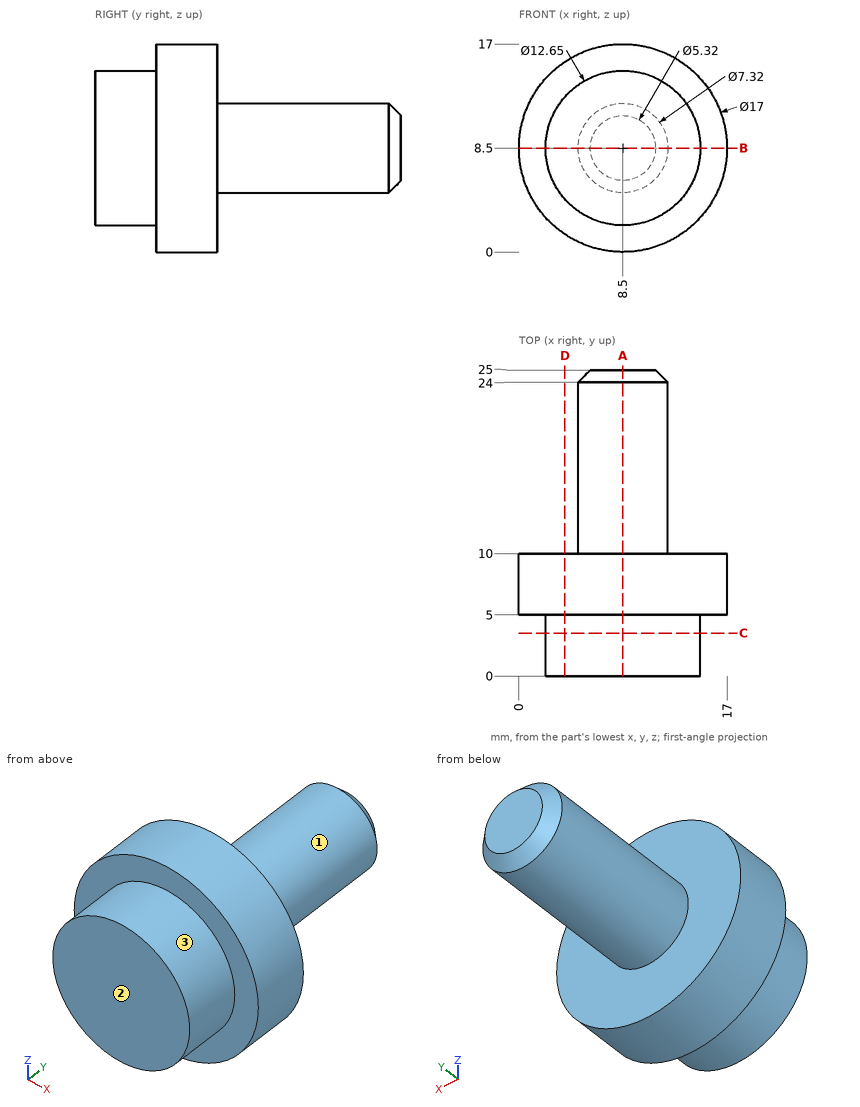
Print and shaded views of the part. All mm, measured from the part's lowest x, y and z. A direction names the side the tool comes from. Round coordinates to 2 decimals unless told otherwise and drop trailing zeros. Write each loop counter-clockwise with the first axis right and the second up, starting at its lowest first coordinate (ties: lowest second). Pieces come first, ordered by that corner, then holes. Notation, with made-up numbers: (46, -13.75) - (59, -13.75) arc R24 cw to (59, -2.75) - close; hole circle Ø1 at (1, 33.5). An arc over 180 degrees is marked (long way). Use CSV: the item, a comma, the result in double quotes. Start each with the question number.
Item 1: Band-saw the part on B-B (z = 8.5). Write the cut outline in (x, y) (3 decimals).
Item 2: Band-saw the part on A-A (x = 8.5). Write the cut outline in (y, z) (3 decimals).
Item 3: Tool access for the marked faces 1, 2 and 3: list every direction of +Z, -Z, +X, -X, +Y, -Y with a clear straight run to the whole face (end or side of a thin tool).
Item 4: Band-saw the part on C-C (y = 3.5). Write the cut outline in (x, z) (3 decimals).
Item 5: Pin check, flat tips, straight feed: P1, Ø1.5, axis at x = 15, z = 14.5, coming from the +Y side; P2, Ø10, axis at x = 4, z = 2, coming from the -Y side; P3, Ø1.5, axis at x = 14.5, y = 5, coming from the -Z side; P4, Ø10, axis at x = 6, y = 22.5, coming from the +Z side. Stop position of each tip, or through.
Item 6: Drill centre lines: L1, parallel to Y at x = 11, z = 5.25; L2, parallel to Y at x = 16, z = 7.75; L3, parallel to Z at x = 6.5, y = 7.25. Where is each one in solid material? Low to high. Write a range as [from, to].
Item 7: Band-saw the part on D-D (x = 3.75). Write the cut outline in (y, z).
Checked values:
1,outline,"(0, 5) - (2.175, 5) - (2.175, 0) - (14.825, 0) - (14.825, 5) - (17, 5) - (17, 10) - (12.16, 10) - (12.16, 24) - (11.16, 25) - (5.84, 25) - (4.84, 24) - (4.84, 10) - (0, 10) - close"
2,outline,"(0, 2.175) - (5, 2.175) - (5, 0) - (10, 0) - (10, 4.84) - (24, 4.84) - (25, 5.84) - (25, 11.16) - (24, 12.16) - (10, 12.16) - (10, 17) - (5, 17) - (5, 14.825) - (0, 14.825) - close"
3,face 1,"+Y"
3,face 2,"+Z, -Z, +X, -X, -Y"
3,face 3,"-Y"
4,outline,"circle Ø12.65 at (8.5, 8.5)"
5,P1,"stops at y = 10"
5,P2,"stops at y = 0"
5,P3,"stops at z = 1.82"
5,P4,"stops at z = 12.16"
6,L1,"y = [0, 10]"
6,L2,"y = [5, 10]"
6,L3,"z = [0.24, 16.76]"
7,outline,"(0, 4.32) - (5, 4.32) - (5, 1.45) - (10, 1.45) - (10, 15.55) - (5, 15.55) - (5, 12.68) - (0, 12.68) - close"
